from build123d import *

# Parameters (mm, degrees)
BOSS_EXTRUDE1_DEPTH = 9.525
SKETCH6_R           = 1.905
CUT_EXTRUDE2_DEPTH  = 25.46325319
SKETCH7_R           = 1.905
CUT_EXTRUDE3_DEPTH  = 25.464227008
FILLET1_R           = 0.79375


with BuildPart() as part:
    # Sketch1 → Boss-Extrude1 (new, symmetric)
    with BuildSketch(Plane.XY):
        Polygon((-5.755049727, -1.093010514), (-6.085429683, 21.348472195), (-4.035272706, 21.696550963), (0, 0), align=None)
    extrude(amount=BOSS_EXTRUDE1_DEPTH, both=True)

    # Sketch6 → Cut-Extrude2 (cut, through all)
    with BuildSketch(Plane(origin=(-5.769890331, -0.084943412, 0), x_dir=(0, 0, 1), z_dir=(-0.9998916512998705, -0.014720246628988168, 0))):
        with Locations(Location((-4.7625, 3.863780902, 0), (0, 0, 270))):
            Circle(SKETCH6_R)
        with Locations(Location((-4.7625, 16.563780902, 0), (0, 0, 270))):
            Circle(SKETCH6_R)
    extrude(amount=-CUT_EXTRUDE2_DEPTH, mode=Mode.SUBTRACT)

    # Sketch7 → Cut-Extrude3 (cut, through all)
    with BuildSketch(Plane(origin=(0, 0, 0), x_dir=(0, 0, -1), z_dir=(0.9831405992384419, 0.18285120215376635, 0))):
        with Locations(Location((-5.378603812, 4.71861458, 0), (0, 0, 90))):
            Circle(SKETCH7_R)
    extrude(amount=-CUT_EXTRUDE3_DEPTH, mode=Mode.SUBTRACT)

    # Fillet1
    fillet1_edges = [part.edges().sort_by_distance(p)[0] for p in [
        (-5.060351194, 21.522511579, 9.525),
        (-5.920239705, 10.12773084, 9.525),
        (-2.877524863, -0.546505257, 9.525),
        (-5.920239705, 10.12773084, -9.525),
        (-5.060351194, 21.522511579, -9.525),
        (-2.017636353, 10.848275481, -9.525),
        (-2.877524863, -0.546505257, -9.525),
        (-5.755049727, -1.093010514, 0),
        (-6.085429683, 21.348472195, 0),
        (-4.035272706, 21.696550963, 0),
        (0, 0, 0),
        (-2.017636353, 10.848275481, 9.525),
    ]]
    fillet(fillet1_edges, radius=FILLET1_R)


solid = part.part
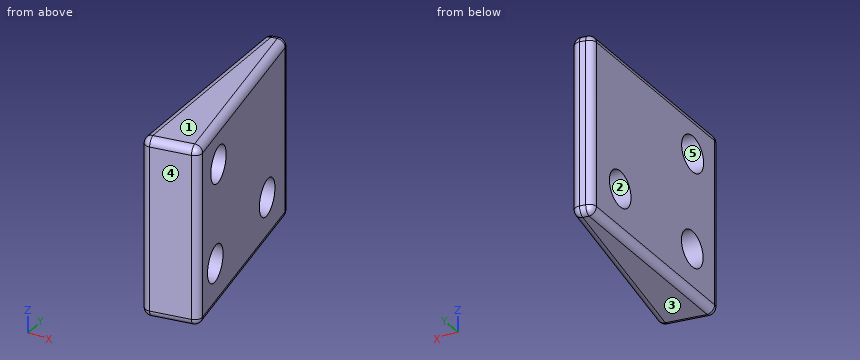
The listing builds one solid part. Answer for the finished solid, in the listing's coordinates (mm). Face numbers are marked on the shaded views. A direction names the side the tool comes from. Give positions to 0.01 mm unless a question says otherwise; leave off trailing zeros. Order: outer loops, then holes, each group sorted by start corner. A loop starts at its lowest first (then second) coordinate and runs counter-clockwise, first axis right, second up. Notation, with made-up numbers: (82.25, 61) - (101.25, 61) arc R20 cw to (101.25, 70) - close; hole circle Ø3 at (17.5, -33). An arc over 180 degrees is marked (long way). Answer as CSV lines item,"result".
Q1. Each of these flat-tipped pins is pushed along its axis until it touches: pin 1 Ø5 at (y, z) = (6, 7.5) entering from -X; pin 2 Ø8 at (y, z) = (15.5, 3) entering from -X; pin 3 Ø3 at (y, z) = (14.5, 3) entering from -X. Where does it stop, or does it pass through?
Answer key:
pin 1,"stops at x = -5.9"
pin 2,"stops at x = -6.06"
pin 3,"stops at x = -6.01"
Q2. A cutting plane is placed at C-C, the plane z = -6. Determine the outline of the cut face in (x, y), and give its area (3 significant figures).
Answer key:
outline,"(-6.08, 20.67) - (-6.04, 17.93) - (-3.34, 17.96) - (-3.89, 20.93) arc R0.79 ccw to (-4.81, 21.57) - (-5.41, 21.46) arc R0.79 ccw to start; (-5.99, 15.03) - (-5.85, 5.23) - (-0.99, 5.3) - (-2.8, 15.08) - close; (-5.81, 2.33) - (-5.77, -0.15) arc R0.79 ccw to (-4.83, -0.92) - (-0.78, -0.15) arc R0.79 ccw to (-0.14, 0.78) - (-0.45, 2.41) - close"
area,"63.8 mm^2"
Q3. A cutting plane is placed at D-D, the plane x = -3.3. Count the separate pieces of the cut face and the enclosed holes in it, and give its area (3 significant figures).
Answer key:
separate pieces,"1"
enclosed holes,"2"
area,"315 mm^2"
Q4. Determine the mould class of the marked faces 3, 4 and 5 for opening direction Y: pulls with the +Y half, pulls with the -Y half, needs draft (parallel to the pull), parting line crosses it, or undercut.
Answer key:
face 3,"needs draft"
face 4,"pulls with the -Y half"
face 5,"undercut"
Q5. Which of the six approach directions +Z, -Z, +X, -X, +Y, -Y give full straight-line access (tool end or side, diameter ignored) to the marked faces 1 and 2?
Answer key:
face 1,"+Z, +X, -X, +Y, -Y"
face 2,"none"
Q6. A cutting plane is placed at A-A, the plane z = 4.25. Determine the outline of the cut face in (x, y), and give its area (3 significant figures).
Answer key:
outline,"(-6.08, 20.67) - (-5.85, 5.27) - (-1.14, 6.15) - (-3.89, 20.93) arc R0.79 ccw to (-4.81, 21.57) - (-5.41, 21.46) arc R0.79 ccw to start; (-5.8, 2.16) - (-5.77, -0.15) arc R0.79 ccw to (-4.83, -0.92) - (-0.78, -0.15) arc R0.79 ccw to (-0.14, 0.78) - (-0.58, 3.13) - close"
area,"71.6 mm^2"
Q7. A cutting plane is placed at B-B, the plane z = 8. Determine the outline of the cut face in (x, y).
Answer key:
outline,"(-6.08, 20.67) - (-5.77, -0.15) arc R0.79 ccw to (-4.83, -0.92) - (-0.78, -0.15) arc R0.79 ccw to (-0.14, 0.78) - (-3.89, 20.93) arc R0.79 ccw to (-4.81, 21.57) - (-5.41, 21.46) arc R0.79 ccw to start"
Q8. Straight lines are drawn through the part: L1, parallel to Z at x = -4.4, y = 16.5 (1 decimal); L2, parallel to Y at x = -5.65, z = -5.5; L3, parallel to Z at x = -4.2, y = 4.75 (3 decimals). For each, find the intervals that lie inside material, in ascending order.
Answer key:
L1,"z = -9.5 to -6.7, -2.9 to 9.5"
L2,"y = -0.56 to 2.02, 5.54 to 14.73, 18.24 to 21.38"
L3,"z = -9.525 to -6.415, -3.11 to 3.615, 7.143 to 9.525"
